Check sheet for the drawn part. Datum: minimum x, y, z corner. Units: mm. A direction names the side the tool comes from. Give positions to 0.01 mm unless a question says otherwise; leave off trailing zeros. Loops run counter-clockwise (first coordinate to the right, second up) from the corner with the lowest first, then second, coordinate; pieces in that order, holes last. Notation, with made-up numbers: (33.25, 51) - (78.25, 51) arc R28 ccw to (78.25, 85) - close; hole circle Ø7 at (0, -22.75). An arc over 180 degrees is marked (long way). Use one line per item in the form item = value.
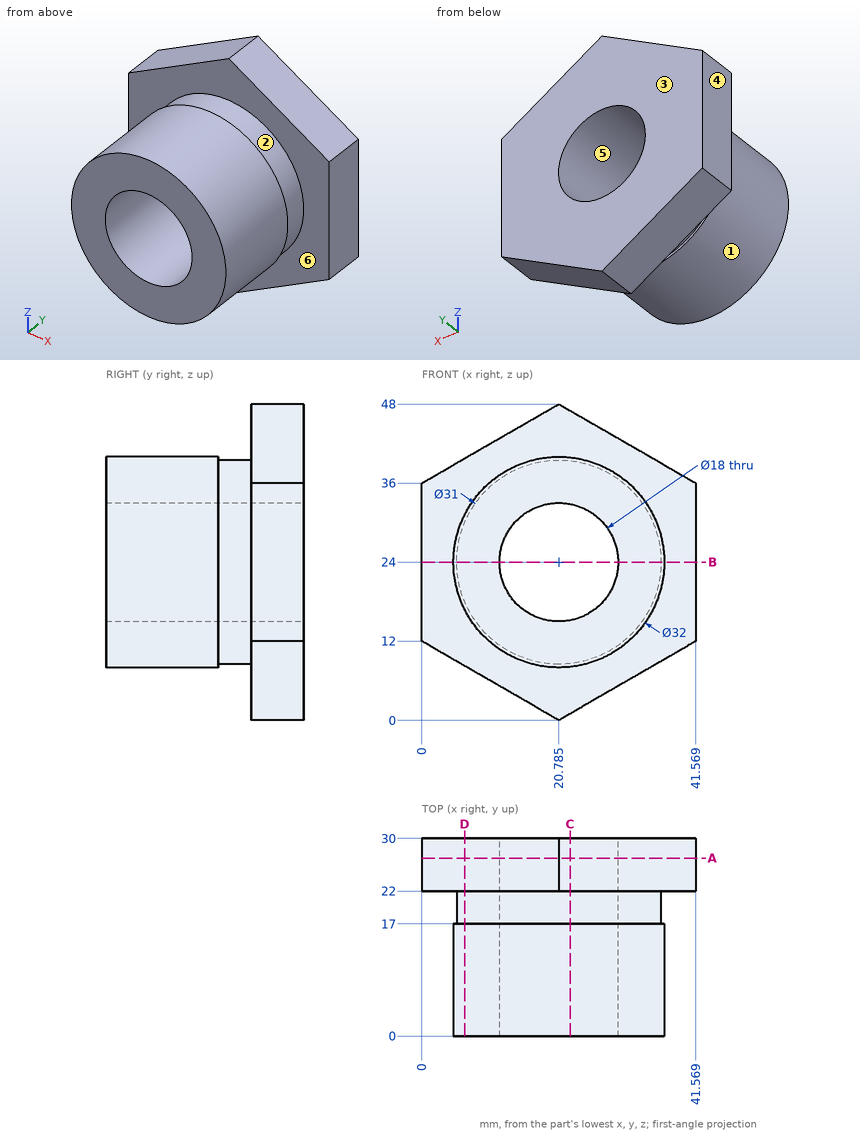
Item 1: Section check A-A on y = 27. Record the boundary of the cut face in (x, z) (1 decimal).
Answer block:
outline = (0, 12) - (20.8, 0) - (41.6, 12) - (41.6, 36) - (20.8, 48) - (0, 36) - close; hole circle Ø18 at (20.8, 24)
Item 2: Section check D-D on x = 6.5. Record the boundary of the cut face in (y, z).
Answer block:
outline = (0, 16.79) - (17, 16.79) - (17, 17.98) - (22, 17.98) - (22, 8.25) - (30, 8.25) - (30, 39.75) - (22, 39.75) - (22, 30.02) - (17, 30.02) - (17, 31.21) - (0, 31.21) - close
Item 3: Thickness scan on L1, parallel to X at y = 23, z = 24 (1 decimal); L2, parallel to X at y = 20.5, z = 24 (1 decimal); L3, parallel to Y at x = 23.5, z = 7.5. Record the ranges inside material, lowest first.
Answer block:
L1 = 0 to 11.8, 29.8 to 41.6
L2 = 5.3 to 11.8, 29.8 to 36.3
L3 = 22 to 30
Item 4: Section check B-B on z = 24. Record the boundary of the cut face in (x, y) (1 decimal).
Answer block:
outline = (0, 22) - (5.3, 22) - (5.3, 17) - (4.8, 17) - (4.8, 0) - (11.8, 0) - (11.8, 30) - (0, 30) - close; (29.8, 0) - (36.8, 0) - (36.8, 17) - (36.3, 17) - (36.3, 22) - (41.6, 22) - (41.6, 30) - (29.8, 30) - close
Item 5: Mould release check, pull along X, two halves, no side actions. Record for the marked faces 4, 5 and 6: released by +X, released by -X, zero draft, split by the parting line, or undercut.
Answer block:
face_4 = released by -X
face_5 = undercut
face_6 = zero draft
Item 6: Access from +Z, -Z, +X, -X, +Y, -Y to the whole of each face (thin tool, end or side, straight path). Record for the marked faces 1, 2 and 3.
Answer block:
face_1 = -Y
face_2 = none
face_3 = +Z, -Z, +X, -X, +Y
Item 7: Section check C-C on x = 22.5. Record the boundary of the cut face in (y, z) (1 decimal).
Answer block:
outline = (0, 8.1) - (17, 8.1) - (17, 8.6) - (22, 8.6) - (22, 1) - (30, 1) - (30, 15.2) - (0, 15.2) - close; (0, 32.8) - (30, 32.8) - (30, 47) - (22, 47) - (22, 39.4) - (17, 39.4) - (17, 39.9) - (0, 39.9) - close
Item 8: Gauge pin test, flat ends, axial feed: P1, Ø3, axis at y = 18.5, z = 38, coming from the +X side; P2, Ø1.5, axis at x = 23.5, y = 10.5, coming from the -Z side; P3, Ø5, axis at y = 5, z = 21.5, coming from the -X side (1 decimal). Record the tip position at first contact, or that the pin passes through.
Answer block:
P1 = 29.95
P2 = 8.12
P3 = 4.8
